Check sheet for the modelled part. Datum: model origin and axes. Units: mm. Round coordinates to 2 decimals unless told otherwise and drop trailing zeros. Order: outer loops, then holes, each group sorted by start corner. A loop starts at its lowest first (then second) coordinate and runs counter-clockwise, first axis right, second up.
```python
from build123d import *

# Parameters (mm, degrees)
SKETCH_2_W          = 10
SKETCH_2_H          = 10
SKETCH_2_W_2        = 8
SKETCH_2_H_2        = 8
EXTRUDE_1_DEPTH     = 100
SKETCH_3_R          = 1.6
CUT_EXTRUDE_1_DEPTH = 101.623058987
SKETCH_4_R          = 1.6
CUT_EXTRUDE_2_DEPTH = 101.623058987
SKETCH_7_R          = 1.6
CUT_EXTRUDE_4_DEPTH = 101.623058987


with BuildPart() as part:
    # ｽｹｯﾁ2 → 押し出し-薄板1 (new body)
    with BuildSketch(Plane.XY):
        Rectangle(SKETCH_2_W, SKETCH_2_H)
        Rectangle(SKETCH_2_W_2, SKETCH_2_H_2, mode=Mode.SUBTRACT)
    extrude(amount=EXTRUDE_1_DEPTH)

    # ｽｹｯﾁ3 → ｶｯﾄ - 押し出し1 (cut, through all)
    with BuildSketch(Plane(origin=(5, 0, 0), x_dir=(0, 0, -1), z_dir=(1, 0, 0))):
        with Locations(Location((-95, 0, 0), (0, 0, 90))):
            Circle(SKETCH_3_R)
        with Locations(Location((-5, 0, 0), (0, 0, 270))):
            Circle(SKETCH_3_R)
        with Locations(Location((-40, 0, 0), (0, 0, 90))):
            Circle(SKETCH_3_R)
    extrude(amount=-CUT_EXTRUDE_1_DEPTH, mode=Mode.SUBTRACT)

    # ｽｹｯﾁ4 → ｶｯﾄ - 押し出し2 (cut, through all)
    with BuildSketch(Plane(origin=(0, 5, 0), x_dir=(1, 0, 0), z_dir=(0, 1, 0))):
        with Locations(Location((0, -15, 0), (0, 0, 180))):
            Circle(SKETCH_4_R)
    extrude(amount=-CUT_EXTRUDE_2_DEPTH, mode=Mode.SUBTRACT)

    # ｽｹｯﾁ7 → ｶｯﾄ - 押し出し4 (cut, through all)
    with BuildSketch(Plane(origin=(0, 5, 0), x_dir=(1, 0, 0), z_dir=(0, 1, 0))):
        with Locations(Location((0, -85, 0), (0, 0, 180))):
            Circle(SKETCH_7_R)
    extrude(amount=-CUT_EXTRUDE_4_DEPTH, mode=Mode.SUBTRACT)


solid = part.part
```
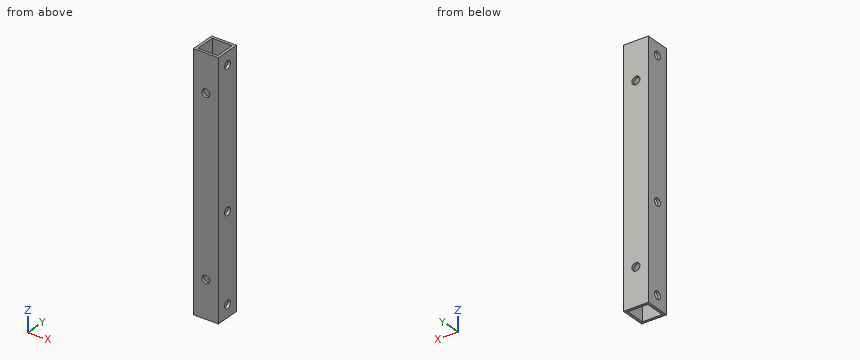
Item 1: Scan lines: line 1 along Z through (x, y) = (-4.5, 0); line 2 along Y through (x, z) = (-4.55, 95); line 3 along X through (y, z) = (2.5, 71.5). Record each from-to range of solid material in increasing order.
Answer:
line 1: z = 0 to 3.4, 6.6 to 38.4, 41.6 to 93.4, 96.6 to 100
line 2: y = -5 to -1.6, 1.6 to 5
line 3: x = -5 to -4, 4 to 5
Item 2: Go/stop test with a flat-tipped pin: P1, Ø2.5, axis at y = 0, z = 95, coming from the +X side. Record where the tip stops, or that it passes through.
Answer:
P1: passes through
Item 3: Sectioned sample at D-D (z = 74.5). Record the cut outline in (x, y).
Answer:
outline: (-5, -5) - (5, -5) - (5, 5) - (-5, 5) - close; hole (-4, -4) - (4, -4) - (4, 4) - (-4, 4) - close
Item 4: Sectioned sample at A-A (y = -3). Record the cut outline in (x, z), and give its area (3 significant figures).
Answer:
outline: (-5, 0) - (-4, 0) - (-4, 100) - (-5, 100) - close; (4, 0) - (5, 0) - (5, 100) - (4, 100) - close
area: 200 mm2
Item 5: Sectioned sample at B-B (z = 95). Record the cut outline in (x, y).
Answer:
outline: (-5, -5) - (5, -5) - (5, -1.6) - (4, -1.6) - (4, -4) - (-4, -4) - (-4, -1.6) - (-5, -1.6) - close; (-5, 1.6) - (-4, 1.6) - (-4, 4) - (4, 4) - (4, 1.6) - (5, 1.6) - (5, 5) - (-5, 5) - close
Item 6: Sectioned sample at C-C (x = 0). Record the cut outline in (y, z).
Answer:
outline: (-5, 0) - (-4, 0) - (-4, 13.4) - (-5, 13.4) - close; (-5, 16.6) - (-4, 16.6) - (-4, 83.4) - (-5, 83.4) - close; (-5, 86.6) - (-4, 86.6) - (-4, 100) - (-5, 100) - close; (4, 0) - (5, 0) - (5, 13.4) - (4, 13.4) - close; (4, 16.6) - (5, 16.6) - (5, 83.4) - (4, 83.4) - close; (4, 86.6) - (5, 86.6) - (5, 100) - (4, 100) - close
